Check sheet for the drawn part. Datum: minimum x, y, z corner. Units: mm. A direction names the side the tool comes from. Coordinates: 2 decimals unless noted, no trailing zeros. Loops run counter-clockwise (first coordinate to the right, second up) from the corner with the lowest first, then second, coordinate; pieces in that order, holes last.
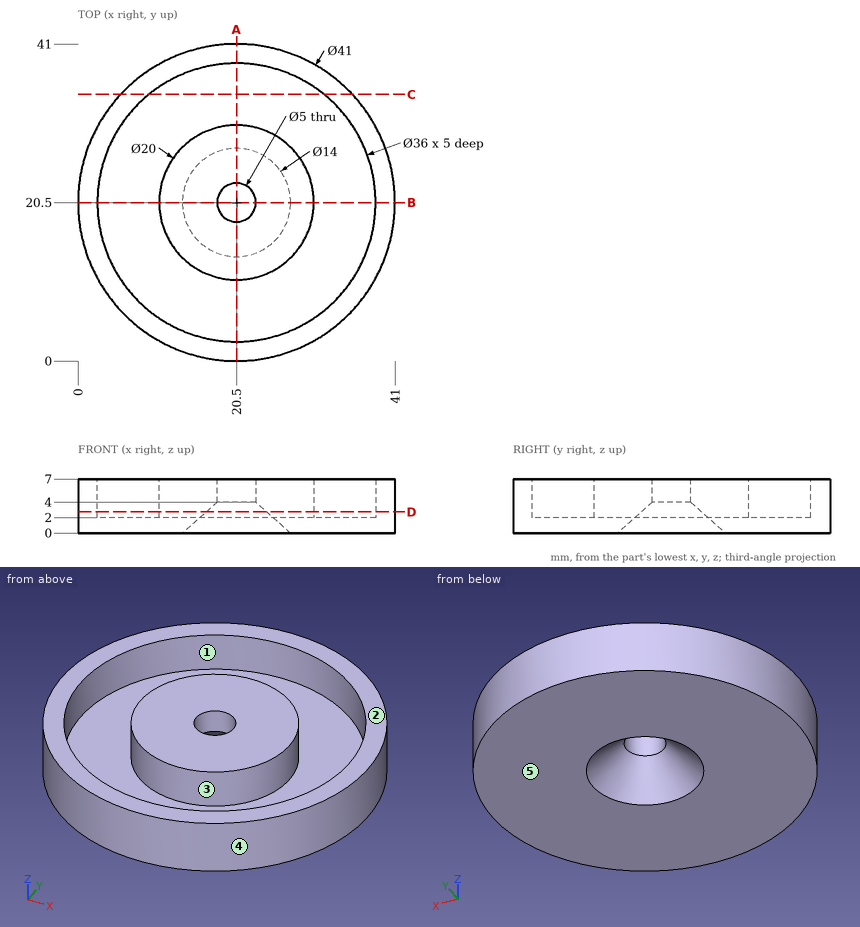
(1) Sectioned sample at D-D on z = 2.75. Record the cut outline in (x, y).
Findings:
outline: circle Ø41 at (20.5, 20.5); circle Ø20 at (20.5, 20.5); hole circle Ø36 at (20.5, 20.5); hole circle Ø7.81 at (20.5, 20.5)
(2) Gauge pin test, flat ends, axial feed: pin 1 Ø1 at (y, z) = (35, 6) entering from -X (3 decimals); pin 2 Ø4 at (x, z) = (4.5, 4.5) entering from -Y (3 decimals); pin 3 Ø1 at (x, z) = (17, 3.5) entering from -Y. Record the tip position at first contact, or that the pin passes through.
Findings:
pin 1: stops at x = 5.525
pin 2: stops at y = 5.525
pin 3: stops at y = 0.22
(3) Sectioned sample at C-C on y = 34.5. Record the cut outline in (x, z), and give its area (3 significant figures).
Findings:
outline: (5.53, 0) - (35.47, 0) - (35.47, 7) - (31.81, 7) - (31.81, 2) - (9.19, 2) - (9.19, 7) - (5.53, 7) - close
area: 96.5 mm2
(4) Draft check along X on the marked faces 3, 4 and 5. Enter one of: +X half, -X half, draft (parallel to the pull), parting line (faces both ways), or undercut.
Findings:
face 3: undercut
face 4: parting line
face 5: draft
(5) Sectioned sample at A-A on x = 20.5. Record the cut outline in (y, z), and give its area (3 significant figures).
Findings:
outline: (0, 0) - (13.5, 0) - (18, 4) - (18, 7) - (10.5, 7) - (10.5, 2) - (2.5, 2) - (2.5, 7) - (0, 7) - close; (23, 4) - (27.5, 0) - (41, 0) - (41, 7) - (38.5, 7) - (38.5, 2) - (30.5, 2) - (30.5, 7) - (23, 7) - close
area: 154 mm2
(6) Access from +Z, -Z, +X, -X, +Y, -Y to the whole of each face (thin tool, end or side, straight path). Record for the marked faces 1 and 2.
Findings:
face 1: +Z
face 2: +Z, +X, -X, +Y, -Y
(7) Scan lines: L1, parallel to Y at x = 20.5, z = 4.9; L2, parallel to X at y = 28, z = 5.75; L3, parallel to Y at x = 16.5, z = 2.25. Record each from-to range of solid material in increasing order.
Findings:
L1: y = 0 to 2.5, 10.5 to 18, 23 to 30.5, 38.5 to 41
L2: x = 1.42 to 4.14, 13.89 to 27.11, 36.86 to 39.58
L3: y = 0.39 to 2.95, 11.33 to 18.51, 22.49 to 29.67, 38.05 to 40.61
